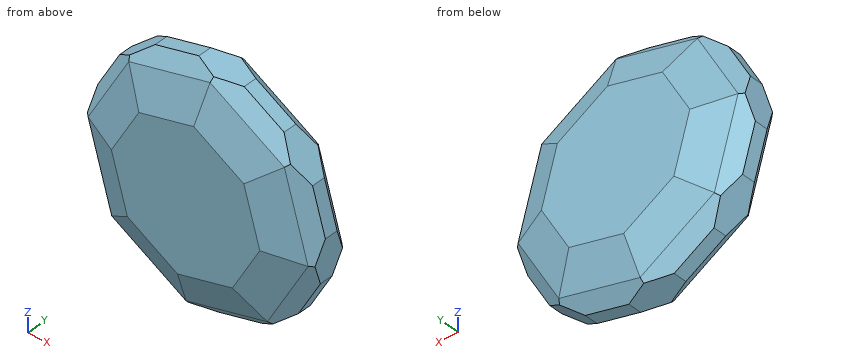
```python
from build123d import *

# Parameters (mm, degrees)
F1_DEPTH = 25.4
F2_SIZE  = 10.16
F3_SIZE  = 7.62
F4_SIZE  = 7.62
F5_SIZE  = 10.16
F6_SIZE  = 7.62


with BuildPart() as f1:
    # F0 (on Front) → F1 (new body)
    with BuildSketch(Plane.XZ):
        Polygon((40.479728647, 21.0820164172), (29.3306543749, 34.9681649717), (13.7162538572, 43.5307273965), (-3.986321972, 45.4661311822), (-21.0820164172, 40.479728647), (-34.9681649717, 29.3306543749), (-43.5307273965, 13.7162538572), (-45.4661311822, -3.986321972), (-40.479728647, -21.0820164172), (-29.3306543749, -34.9681649717), (-13.7162538572, -43.5307273965), (3.986321972, -45.4661311822), (21.0820164172, -40.479728647), (34.9681649717, -29.3306543749), (43.5307273965, -13.7162538572), (45.4661311822, 3.986321972), align=None)
    extrude(amount=F1_DEPTH)

    # F2 (call 1 of 8: OpenCascade refuses the feature's edges together)
    f2_edges = [f1.edges().sort_by_distance(p)[0] for p in [
        (39.249446, -25.4, -21.523454),
    ]]
    chamfer(f2_edges, length=F2_SIZE)

    # F2#2 (call 2 of 8)
    f2_2_edges = [f1.edges().sort_by_distance(p)[0] for p in [
        (42.97293, -25.4, 12.534169),
    ]]
    chamfer(f2_2_edges, length=F2_SIZE)

    # F2#3 (call 3 of 8)
    f2_3_edges = [f1.edges().sort_by_distance(p)[0] for p in [
        (21.523454, -25.4, 39.249446),
    ]]
    chamfer(f2_3_edges, length=F2_SIZE)

    # F2#4 (call 4 of 8)
    f2_4_edges = [f1.edges().sort_by_distance(p)[0] for p in [
        (-12.534169, -25.4, 42.97293),
    ]]
    chamfer(f2_4_edges, length=F2_SIZE)

    # F2#5 (call 5 of 8)
    f2_5_edges = [f1.edges().sort_by_distance(p)[0] for p in [
        (-39.249446, -25.4, 21.523454),
    ]]
    chamfer(f2_5_edges, length=F2_SIZE)

    # F2#6 (call 6 of 8)
    f2_6_edges = [f1.edges().sort_by_distance(p)[0] for p in [
        (-42.97293, -25.4, -12.534169),
    ]]
    chamfer(f2_6_edges, length=F2_SIZE)

    # F2#7 (call 7 of 8)
    f2_7_edges = [f1.edges().sort_by_distance(p)[0] for p in [
        (-21.523454, -25.4, -39.249446),
    ]]
    chamfer(f2_7_edges, length=F2_SIZE)

    # F2#8 (call 8 of 8)
    f2_8_edges = [f1.edges().sort_by_distance(p)[0] for p in [
        (12.534169, -25.4, -42.97293),
    ]]
    chamfer(f2_8_edges, length=F2_SIZE)

    # F3
    f3_edges = [f1.edges().sort_by_distance(p)[0] for p in [
        (-30.34099, -25.4, 16.638271),
        (16.638271, -25.4, 30.34099),
        (30.34099, -25.4, -16.638271),
        (-16.638271, -25.4, -30.34099),
    ]]
    chamfer(f3_edges, length=F3_SIZE)

    # F4
    f4_edges = [f1.edges().sort_by_distance(p)[0] for p in [
        (-9.689286, -25.4, 33.219354),
        (33.219354, -25.4, 9.689286),
        (9.689286, -25.4, -33.219354),
        (-33.219354, -25.4, -9.689286),
    ]]
    chamfer(f4_edges, length=F4_SIZE)

    # F5 (call 1 of 8: OpenCascade refuses the feature's edges together)
    f5_edges = [f1.edges().sort_by_distance(p)[0] for p in [
        (-21.523454, 0, -39.249446),
    ]]
    chamfer(f5_edges, length=F5_SIZE)

    # F5#2 (call 2 of 8)
    f5_2_edges = [f1.edges().sort_by_distance(p)[0] for p in [
        (12.534169, 0, -42.97293),
    ]]
    chamfer(f5_2_edges, length=F5_SIZE)

    # F5#3 (call 3 of 8)
    f5_3_edges = [f1.edges().sort_by_distance(p)[0] for p in [
        (39.249446, 0, -21.523454),
    ]]
    chamfer(f5_3_edges, length=F5_SIZE)

    # F5#4 (call 4 of 8)
    f5_4_edges = [f1.edges().sort_by_distance(p)[0] for p in [
        (42.97293, 0, 12.534169),
    ]]
    chamfer(f5_4_edges, length=F5_SIZE)

    # F5#5 (call 5 of 8)
    f5_5_edges = [f1.edges().sort_by_distance(p)[0] for p in [
        (21.523454, 0, 39.249446),
    ]]
    chamfer(f5_5_edges, length=F5_SIZE)

    # F5#6 (call 6 of 8)
    f5_6_edges = [f1.edges().sort_by_distance(p)[0] for p in [
        (-12.534169, 0, 42.97293),
    ]]
    chamfer(f5_6_edges, length=F5_SIZE)

    # F5#7 (call 7 of 8)
    f5_7_edges = [f1.edges().sort_by_distance(p)[0] for p in [
        (-39.249446, 0, 21.523454),
    ]]
    chamfer(f5_7_edges, length=F5_SIZE)

    # F5#8 (call 8 of 8)
    f5_8_edges = [f1.edges().sort_by_distance(p)[0] for p in [
        (-42.97293, 0, -12.534169),
    ]]
    chamfer(f5_8_edges, length=F5_SIZE)

    # F6
    f6_edges = [f1.edges().sort_by_distance(p)[0] for p in [
        (16.638271, 0, 30.34099),
        (-9.689286, 0, 33.219354),
        (-30.34099, 0, 16.638271),
        (-33.219354, 0, -9.689286),
        (-16.638271, 0, -30.34099),
        (9.689286, 0, -33.219354),
        (30.34099, 0, -16.638271),
        (33.219354, 0, 9.689286),
    ]]
    chamfer(f6_edges, length=F6_SIZE)


solid = f1.part
```
Geometry check sheet. Reference: the model listing, model coordinates, mm. Coordinates: 2 decimals unless noted, no trailing zeros. Write each loop counter-clockwise with the first axis right and the second up, starting at its lowest first coordinate (ties: lowest second). Pieces come first, ordered by that corner, then holes. Notation, with made-up numbers: (32.25, 5) -> (54.25, 5) arc R27 cw to (54.25, 40) -> close; hole circle Ø4 at (-28.75, 10.25). An arc over 180 degrees is marked (long way). Use CSV: the item, a comma, the result in double quotes. Start each with the question number.
Item 1: Depth check by flat-ended pin: pin 1 Ø4 at (x, y) = (-27.5, -21) entering from +Z; pin 2 Ø12 at (x, z) = (-29, -12.5) entering from +Y; pin 3 Ø8 at (x, z) = (-19, 28) entering from +Y; pin 4 Ø5 at (y, z) = (-19, 0.5) entering from +X. Enter the tip coordinate at first touch or a pass-through.
Item 2: Thickness scan on line 1 (Z direction, x = 31, y = -8); line 2 (Y direction, x = 19, z = -25.5); line 3 (Z direction, x = 26, y = -5.75). Record the ranges inside material, lowest first.
Item 3: Cross-section at C-C, the plane x = 12. Record the cut outline in (y, z), plus the area to 3 significant figures.
Item 4: Cross-section at B-B, the plane z = -25.5. Record the cut outline in (x, y), plus the area to 3 significant figures.
Item 5: Cross-section at A-A, the plane y = -13. Record the cut outline in (x, z).
Item 6: Cross-section at D-D, the plane z = -7.5. Record the cut outline in (x, y).
Answers:
1,pin 1,"z = 34.77"
1,pin 2,"y = 0"
1,pin 3,"y = -0.5"
1,pin 4,"x = 45.11"
2,line 1,"-32.07 to 31.59"
2,line 2,"-24.23 to -1.17"
2,line 3,"-34.45 to 31.77"
3,outline,"(-25.4, -24.61) -> (-20.01, -38.16) -> (-15.24, -43.13) -> (-10.16, -43.13) -> (-5.39, -38.16) -> (0, -24.61) -> (0, 24.19) -> (-5.39, 39.03) -> (-9.5, 43.72) -> (-15.9, 43.72) -> (-20.01, 39.03) -> (-25.4, 24.19) -> close"
3,area,"1,910 mm^2"
4,outline,"(-36.93, -17.41) -> (-34.22, -20.01) -> (-31.76, -20.99) -> (-9.62, -25.4) -> (8.94, -25.4) -> (20.47, -24.06) -> (31.63, -20.01) -> (37.07, -15.24) -> (37.07, -10.16) -> (31.63, -5.39) -> (20.47, -1.34) -> (8.94, 0) -> (-9.62, 0) -> (-31.76, -4.41) -> (-34.22, -5.39) -> (-36.93, -7.99) -> close"
4,area,"1,550 mm^2"
5,outline,"(-45.47, -3.99) -> (-40.48, -21.08) -> (-29.33, -34.97) -> (-13.72, -43.53) -> (3.99, -45.47) -> (21.08, -40.48) -> (34.97, -29.33) -> (43.53, -13.72) -> (45.47, 3.99) -> (40.48, 21.08) -> (29.33, 34.97) -> (13.72, 43.53) -> (-3.99, 45.47) -> (-21.08, 40.48) -> (-34.97, 29.33) -> (-43.53, 13.72) -> close"
6,outline,"(-44.44, -15.24) -> (-39.47, -20.01) -> (-25.92, -25.4) -> (26.66, -25.4) -> (41.5, -20.01) -> (44.21, -17.63) -> (44.21, -7.77) -> (41.5, -5.39) -> (26.66, 0) -> (-25.92, 0) -> (-39.47, -5.39) -> (-44.44, -10.16) -> close"
